from build123d import *

# Parameters (mm, degrees)
CHAMFER2_SIZE       = 7
CHAMFER2_SIZE2      = 1.5
SKETCH2_R           = 11.5
BOSS_EXTRUDE1_DEPTH = 19
SKETCH3_R           = 17
BOSS_EXTRUDE2_DEPTH = 22.5
CHAMFER3_SIZE       = 2
CHAMFER3_SIZE2      = 4
CUT_EXTRUDE1_DEPTH  = 41
CIRPATTERN1_COUNT   = 6
SKETCH21_R          = 40
BOSS_EXTRUDE9_DEPTH = 238


with BuildPart() as part:
    # Sketch1 → Revolve1 (revolve)
    with BuildSketch(Plane(origin=(0, 0, 0), x_dir=(0, 0, -1), z_dir=(1, 0, 0))):
        Polygon((0, 128.3), (0, -128.3), (-24.1, -128.3), (-24.1, -123.7), (-30, -123.7), (-30, -109.7), (-39.9, -109.7), (-39.9, -99.7), (-40, -99.7), (-40, 100.3), (-39.9, 100.3), (-39.9, 128.3), align=None)
    revolve(axis=Axis((0, 128.3, 0), (0, -1, 0)))

    # Chamfer2
    chamfer2_edges = [part.edges().sort_by_distance(p)[0] for p in [
        (0, -128.3, -24.1),
    ]]
    chamfer2_side = [part.faces().sort_by_distance(p)[0] for p in [
        (0, -128.3, 0),
    ]]
    chamfer(chamfer2_edges, length=CHAMFER2_SIZE, length2=CHAMFER2_SIZE2, reference=chamfer2_side[0])

    # Sketch2 → Boss-Extrude1 (add)
    with BuildSketch(Plane.XZ.offset(128.3)):
        Circle(SKETCH2_R)
    extrude(amount=BOSS_EXTRUDE1_DEPTH)

    # Sketch3 → Boss-Extrude2 (add)
    with BuildSketch(Plane.XZ.offset(147.3)):
        Circle(SKETCH3_R)
    extrude(amount=BOSS_EXTRUDE2_DEPTH)

    # Chamfer3
    chamfer3_edges = [part.edges().sort_by_distance(p)[0] for p in [
        (-17, -169.8, 0),
    ]]
    chamfer3_side = [part.faces().sort_by_distance(p)[0] for p in [
        (-17, -158.55, 0),
    ]]
    chamfer(chamfer3_edges, length=CHAMFER3_SIZE, length2=CHAMFER3_SIZE2, reference=chamfer3_side[0])

    # Sketch7 → Cut-Extrude1 (cut, symmetric)
    with BuildSketch(Plane(origin=(0, 0, 0), x_dir=(0, 0, -1), z_dir=(1, 0, 0))):
        Polygon((-29.89327327, -143.30672673), (-15, -158.2), (-15, -177.081282463), (-29.89327327, -177.081282463), align=None)
    cut_extrude1 = extrude(amount=CUT_EXTRUDE1_DEPTH, both=True, mode=Mode.SUBTRACT)

    # CirPattern1: Cut-Extrude1 ×6 about axis
    cirpattern1_axis = Axis((0, 0, 0), (0, 1, 0))
    for i in range(1, CIRPATTERN1_COUNT):
        add(cut_extrude1.rotate(cirpattern1_axis, i * 360 / CIRPATTERN1_COUNT), mode=Mode.SUBTRACT)

    # Sketch21 → Boss-Extrude9 (add)
    with BuildSketch(Plane(origin=(0, 128.3, 0), x_dir=(1, 0, 0), z_dir=(0, 1, 0))):
        Circle(SKETCH21_R)
    extrude(amount=-BOSS_EXTRUDE9_DEPTH)


solid = part.part
The listing builds one solid part. Answer for the finished solid, in the listing's coordinates (mm). A direction names the side the tool comes from. Coordinates: 2 decimals unless noted, no trailing zeros. Write each loop counter-clockwise with the first axis right and the second up, starting at its lowest first coordinate (ties: lowest second). Pieces come first, ordered by that corner, then holes. Notation, with made-up numbers: (19, 81) - (60, 81) arc R21 cw to (60, 105) - close; hole circle Ø3 at (5.25, 65). An arc over 180 degrees is marked (long way). Put each result on its own line as item: value.
1. Flat-ended cylindrical pins translate along their axes: pin 1 Ø8 at (x, y) = (-26.5, 76.5) entering from +Z; pin 2 Ø2 at (y, z) = (-90.5, 26.5) entering from -X; pin 3 Ø6 at (y, z) = (78.5, 26.5) entering from +X. Find the tip coordinate at first contact, or state that the pin passes through.
Answer sheet:
pin 1: stops at z = 33.07
pin 2: stops at x = -30.82
pin 3: stops at x = 32.37
2. Determine the mould class of faces 1 (the face through (4, -128.3, -11)), 2 (the face through (0, -169.8, 0)), 3 (the face through (-16.29, -125.23, -17.76)), 4 (the face through (-1.5, -137.7, 11.4)) for opening direction Y: pulls with the +Y half, pulls with the -Y half, needs draft (parallel to the pull), parting line crosses it, or undercut.
Answer sheet:
face 1: undercut
face 2: pulls with the -Y half
face 3: needs draft
face 4: undercut
3. The part is cut by section B-B on y = -9. Give the vertices of the cut face in (x, z).
Answer sheet:
outline: circle Ø80 at (0, 0)
4. The part is cut by section A-A on x = 0. Give the vertices of the cut face in (y, z), plus the area to 3 significant figures.
Answer sheet:
outline: (-169.8, -13) - (-168.8, -15) - (-158.2, -15) - (-156.2, -17) - (-147.3, -17) - (-147.3, -11.5) - (-128.3, -11.5) - (-128.3, -17.1) - (-126.8, -24.1) - (-123.7, -24.1) - (-123.7, -30) - (-109.7, -30) - (-109.7, -40) - (128.3, -40) - (128.3, 40) - (-109.7, 40) - (-109.7, 30) - (-123.7, 30) - (-123.7, 24.1) - (-126.8, 24.1) - (-128.3, 17.1) - (-128.3, 11.5) - (-147.3, 11.5) - (-147.3, 17) - (-156.2, 17) - (-158.2, 15) - (-168.8, 15) - (-169.8, 13) - close
area: 21,200 mm^2
5. A tool of negligible diameter and unlimited length cuts with its end or side. For faces 5 (the face through (4, -147.3, -11)), 6 (the face through (0, -163, 15)), 7 (the face through (-25, -123.7, 0)), 8 (the face through (-12.934, -163.426, 7.597)), from which of +Z, -Z, +X, -X, +Y, -Y can it reach the whole face along a straight path? Write none if from no direction.
Answer sheet:
face 5: none
face 6: +Z, +X, -X, -Y
face 7: -Y
face 8: +Z, -X, -Y
6. Find the intervals of material crossed by line 1 along Y through (x, z) = (-0.5, -24.5); line 2 along X through (y, z) = (-27.5, -1); line 3 along Y through (x, z) = (15, -33.5), in increasing order. Write a range as from..to.
Answer sheet:
line 1: y = -123.7..128.3
line 2: x = -39.99..39.99
line 3: y = -109.7..128.3
